For this review, take the finished solid that the model builds, in its own axes (mm). Face numbers are marked on the shaded views. A direction names the side the tool comes from. Coordinates: 2 decimals unless noted, no trailing zeros. Loops run counter-clockwise (first coordinate to the right, second up) from the corner with the lowest first, then second, coordinate; pieces in that order, holes last. Notation, with made-up numbers: (26.5, -17) - (46.5, -17) arc R31 cw to (46.5, 11) - close; hole circle Ø6 at (9.25, 79.25). An arc over 180 degrees is marked (long way). Answer as a JSON object with one key per item and string values. Group by question number.
Item 1: We need section A-A (y = 4.5). Give the boundary of the cut face in (x, z), then the cut area to 3 significant figures.
Item 2: We need section B-B (x = -5.5). Give the boundary of the cut face in (y, z), then the cut area to 3 significant figures.
Item 3: We need section D-D (x = 1). Give the boundary of the cut face in (y, z), then the cut area to 3 significant figures.
Item 4: Clearance check with flat-ended pins moving along their axes: pin 1 (0.7 mm diameter, centred on x = 6, z = 7, fed in from +Y); pin 2 (1.5 mm diameter, centred on x = -0.5, y = 18, fed in from -Z); pin 3 (4 mm diameter, centred on y = 8.5, z = 7.5, fed in from -X). State where each tip first meets the part, or that it passes through.
Item 5: Tool access review of the marked faces 5, 6, 7 and 8: name each direction out of +Z, -Z, +X, -X, +Y, -Y from which nothing blocks a thin tool from reaching the whole face with its end or side.
Item 6: To check wall thickness, follow line 1 (Z direction, x = -5.5, y = 7); line 2 (X direction, y = 7.25, z = 20.5); line 3 (Z direction, x = -1, y = 8). State the ranges of each line that lie inside material, in increasing order.
Item 7: Mouldability with a two-part tool opening along Z and no side actions: class the marked faces 1, 2, 3 and 4 as released by +Z, released by -Z, zero draft, split by the parting line, or undercut.
Item 8: We need section C-C (z = -10). Give the boundary of the cut face in (x, y), then the cut area to 3 significant figures.
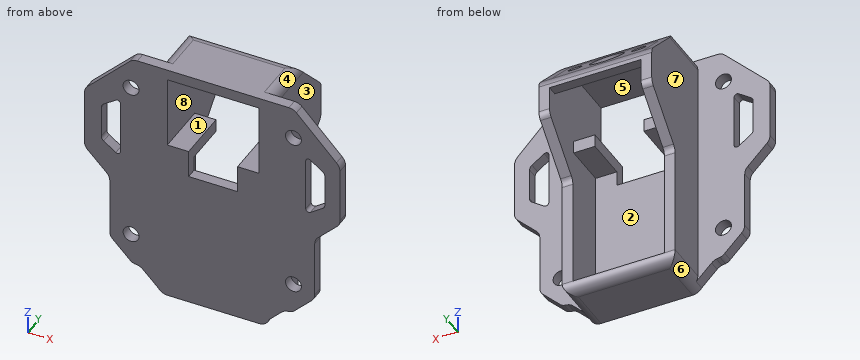
from build123d import *

# Parameters (mm, degrees)
BOSS_EXTRUDE1_DEPTH      = 2
SKETCH2_R                = 1.500000246
SKETCH2_R_2              = 1.5
CUT_EXTRUDE1_DEPTH       = 3
CUT_EXTRUDE3_DEPTH       = 3
SKETCH4_W                = 17.2
SKETCH4_H                = 42.900000423
BOSS_EXTRUDE2_DEPTH      = 16.8
BOSS_EXTRUDE2_DEPTH_BACK = 2
CUT_EXTRUDE4_DEPTH       = 35.442318281
BOSS_EXTRUDE3_REACH      = 34.758
CUT_EXTRUDE5_REACH       = 42.25
SKETCH7_R                = 3.1
SKETCH7_R_2              = 1.3
CUT_EXTRUDE6_REACH       = 4
SKETCH10_W               = 4
SKETCH10_H               = 2.4
BOSS_EXTRUDE4_DEPTH      = 8


with BuildPart() as part:
    # Sketch1 → Boss-Extrude1 (new body)
    with BuildSketch(Plane(origin=(0, 0, 0), x_dir=(1, 0, 0), z_dir=(0, 1, 0))):
        with BuildLine():
            Line((18.572356392, 15.455642083), (15.400781136, 18.627215476))
            ThreePointArc((15.400781136, 18.627215476), (15.000980559, 18.963075341), (14.510830812, 19.14306305))
            Line((14.510830812, 19.14306305), (13.829154841, 19.266075861))
            ThreePointArc((13.829154841, 19.266075861), (13.350450837, 19.465809152), (12.939209066, 19.781927984))
            Line((12.939209066, 19.781927984), (9.538270081, 23.182866969))
            ThreePointArc((9.538270081, 23.182866969), (9.061835297, 23.501210514), (8.499842151, 23.612997901))
            Line((8.499842151, 23.612997901), (-8.368205994, 23.612997901))
            ThreePointArc((-8.368205994, 23.612997901), (-9.221556491, 23.443255933), (-9.94499211, 22.959871707))
            Line((-9.94499211, 22.959871707), (-13.122935832, 19.781927984))
            ThreePointArc((-13.122935832, 19.781927984), (-13.53417801, 19.465808988), (-14.012882539, 19.266075861))
            Line((-14.012882539, 19.266075861), (-14.694557578, 19.14306305))
            ThreePointArc((-14.694557578, 19.14306305), (-15.184706626, 18.963073976), (-15.584504285, 18.627210927))
            Line((-15.584504285, 18.627210927), (-18.756076746, 15.455636602))
            ThreePointArc((-18.756076746, 15.455636602), (-19.189622668, 14.806788967), (-19.341863745, 14.041421099))
            Line((-19.341863745, 14.041421099), (-19.341863745, 3.384570997))
            ThreePointArc((-19.341863745, 3.384570997), (-19.494104434, 2.619205106), (-19.927649253, 1.970359158))
            Line((-19.927649253, 1.970359158), (-23.506077059, -1.608070511))
            ThreePointArc((-23.506077059, -1.608070511), (-23.939622981, -2.25691811), (-24.091864058, -3.022285948))
            Line((-24.091864058, -3.022285948), (-24.091864058, -13.36542942))
            ThreePointArc((-24.091864058, -13.36542942), (-23.939623268, -14.130795551), (-23.506078181, -14.779641628))
            Line((-23.506078181, -14.779641628), (-15.584504285, -22.701215524))
            ThreePointArc((-15.584504285, -22.701215524), (-14.935656966, -23.134761442), (-14.170289369, -23.287002522))
            Line((-14.170289369, -23.287002522), (14.301925526, -23.287002522))
            ThreePointArc((14.301925526, -23.287002522), (15.067293123, -23.134761442), (15.716140442, -22.701215524))
            Line((15.716140442, -22.701215524), (23.23794041, -14.862959876))
            ThreePointArc((23.23794041, -14.862959876), (23.709924747, -14.155388537), (23.90813636, -13.32826184))
            Line((23.90813636, -13.32826184), (23.90813636, -3.022286468))
            ThreePointArc((23.90813636, -3.022286468), (23.755895287, -2.25691839), (23.322349361, -1.608070511))
            Line((23.322349361, -1.608070511), (19.743924908, 1.970357668))
            ThreePointArc((19.743924908, 1.970357668), (19.310378982, 2.619205547), (19.158137909, 3.384573625))
            Line((19.158137909, 3.384573625), (19.158137909, 14.041440986))
            ThreePointArc((19.158137909, 14.041440986), (19.005898249, 14.806801151), (18.572356392, 15.455642083))
        make_face()
    extrude(amount=BOSS_EXTRUDE1_DEPTH)

    # Sketch2 → Cut-Extrude1 (cut, through all)
    with BuildSketch(Plane(origin=(0, 2, 0), x_dir=(1, 0, 0), z_dir=(0, 1, 0))):
        with Locations((-15.341864952, -17.28700247)):
            Circle(SKETCH2_R)
        with Locations((15.158137254, -17.28700247)):
            Circle(SKETCH2_R)
        with Locations((15.158137909, 13.212998804)):
            Circle(SKETCH2_R_2)
        with Locations((-15.341866539, 13.212998804)):
            Circle(SKETCH2_R_2)
    extrude(amount=-CUT_EXTRUDE1_DEPTH, mode=Mode.SUBTRACT)

    # Sketch3 → Cut-Extrude3 (cut, through all)
    with BuildSketch(Plane.XZ):
        with BuildLine():
            Line((18.332290758, 13.738059649), (20.625916482, 12.132045627))
            ThreePointArc((20.625916482, 12.132045627), (20.949257646, 11.763345693), (21.065818079, 11.287002522))
            Line((21.065818079, 11.287002522), (21.065818079, 5.287002522))
            ThreePointArc((21.065818079, 5.287002522), (20.949257646, 4.810659352), (20.625916482, 4.441959417))
            Line((20.625916482, 4.441959417), (18.332290758, 2.835945395))
            ThreePointArc((18.332290758, 2.835945395), (17.762200326, 2.798579694), (17.465818079, 3.287002522))
            Line((17.465818079, 3.287002522), (17.465818079, 13.287002522))
            ThreePointArc((17.465818079, 13.287002522), (17.762200326, 13.77542535), (18.332290758, 13.738059649))
        make_face()
        with BuildLine():
            Line((-17.334181921, 13.287002522), (-17.334181921, 3.287002522))
            ThreePointArc((-17.334181921, 3.287002522), (-17.630564169, 2.798579694), (-18.200654601, 2.835945395))
            Line((-18.200654601, 2.835945395), (-20.494280325, 4.441959417))
            ThreePointArc((-20.494280325, 4.441959417), (-20.817621489, 4.810659352), (-20.934181921, 5.287002522))
            Line((-20.934181921, 5.287002522), (-20.934181921, 11.287002522))
            ThreePointArc((-20.934181921, 11.287002522), (-20.817621489, 11.763345693), (-20.494280325, 12.132045627))
            Line((-20.494280325, 12.132045627), (-18.200654601, 13.738059649))
            ThreePointArc((-18.200654601, 13.738059649), (-17.630564169, 13.77542535), (-17.334181921, 13.287002522))
        make_face()
    extrude(amount=-CUT_EXTRUDE3_DEPTH, mode=Mode.SUBTRACT)

    # Sketch4 → Boss-Extrude2 (add, two sides)
    with BuildSketch(Plane(origin=(0, 2, 0), x_dir=(1, 0, 0), z_dir=(0, 1, 0))) as boss_extrude2_sk:
        with BuildLine():
            Line((-8.534181921, -23.287002522), (8.665818079, -23.287002522))
            ThreePointArc((8.665818079, -23.287002522), (10.080031641, -22.701216085), (10.665818079, -21.287002522))
            Line((10.665818079, -21.287002522), (10.665818079, 21.612997901))
            ThreePointArc((10.665818079, 21.612997901), (10.080031641, 23.027211463), (8.665818079, 23.612997901))
            Line((8.665818079, 23.612997901), (-8.534181921, 23.612997901))
            ThreePointArc((-8.534181921, 23.612997901), (-9.948395484, 23.027211463), (-10.534181921, 21.612997901))
            Line((-10.534181921, 21.612997901), (-10.534181921, -21.287002522))
            ThreePointArc((-10.534181921, -21.287002522), (-9.948395484, -22.701216085), (-8.534181921, -23.287002522))
        make_face()
        with Locations((0.065818079, 0.162997689)):
            Rectangle(SKETCH4_W, SKETCH4_H, mode=Mode.SUBTRACT)
    extrude(amount=BOSS_EXTRUDE2_DEPTH)
    extrude(boss_extrude2_sk.sketch, amount=-BOSS_EXTRUDE2_DEPTH_BACK)

    # Sketch5 → Cut-Extrude4 (cut, through all)
    with BuildSketch(Plane.ZY.offset(10.534181921)):
        with BuildLine():
            Line((-21.612997901, 10.3), (-1.443459743, 10.3))
            ThreePointArc((-1.443459743, 10.3), (-0.676489206, 10.452906013), (-0.026793076, 10.888243804))
            Line((-0.026793076, 10.888243804), (7.271334447, 18.211756196))
            ThreePointArc((7.271334447, 18.211756196), (7.921030577, 18.647093987), (8.688001114, 18.8))
            Line((8.688001114, 18.8), (13.837952846, 18.8))
            ThreePointArc((13.837952846, 18.8), (14.596331781, 18.650638104), (15.2414378, 18.224861392))
            Line((15.2414378, 18.224861392), (22.690487476, 10.887565848))
            ThreePointArc((22.690487476, 10.887565848), (23.131856162, 10.235048322), (23.287002522, 9.462704457))
            Line((23.287002522, 9.462704457), (23.287002522, 6.883402598))
            Line((23.287002522, 6.883402598), (26.098263888, 6.883402598))
            Line((26.098263888, 6.883402598), (26.098263888, 23.771252442))
            Line((26.098263888, 23.771252442), (-26.157105029, 23.771252442))
            Line((-26.157105029, 23.771252442), (-26.157105029, 6.5400194))
            Line((-26.157105029, 6.5400194), (-23.612997901, 6.5400194))
            Line((-23.612997901, 6.5400194), (-23.612997901, 8.3))
            ThreePointArc((-23.612997901, 8.3), (-23.027211463, 9.714213562), (-21.612997901, 10.3))
        make_face()
    extrude(amount=-CUT_EXTRUDE4_DEPTH, mode=Mode.SUBTRACT)

    # Sketch6 → Boss-Extrude3 (add, up to next)
    with BuildSketch(Plane.ZY.offset(-8.665818079), mode=Mode.PRIVATE) as boss_extrude3_sk1:
        with BuildLine():
            Line((21.287002522, 12.269995063), (15.2414378, 18.224861392))
            ThreePointArc((15.2414378, 18.224861392), (14.596331781, 18.650638104), (13.837952846, 18.8))
            Line((13.837952846, 18.8), (13.034792435, 18.8))
            Line((13.034792435, 18.8), (13.034792435, 16.889288371))
            Line((13.034792435, 16.889288371), (21.313555812, 8.73472688))
            Line((21.313555812, 8.73472688), (23.287002522, 8.73472688))
            Line((23.287002522, 8.73472688), (23.287002522, 9.462704457))
            ThreePointArc((23.287002522, 9.462704457), (23.131856162, 10.235048322), (22.690487476, 10.887565848))
            Line((22.690487476, 10.887565848), (21.287002522, 12.269995063))
        make_face()
    boss_extrude3_tool1 = extrude(boss_extrude3_sk1.sketch, amount=BOSS_EXTRUDE3_REACH, mode=Mode.PRIVATE) - part.part
    add(boss_extrude3_tool1.solids().sort_by_distance((8.665818, 13.686528, 18.07587))[0])

    # Sketch7 → Cut-Extrude5 (cut, up to next)
    with BuildSketch(Plane(origin=(0, 16.870013343, 16.6169215), x_dir=(1, 0, 0), z_dir=(0, 0.712430696, 0.701742477)), mode=Mode.PRIVATE) as cut_extrude5_sk1:
        with Locations((0.065818079, -3.297220561)):
            Circle(SKETCH7_R)
    cut_extrude5_tool1 = extrude(cut_extrude5_sk1.sketch, amount=-CUT_EXTRUDE5_REACH, mode=Mode.PRIVATE) & part.part
    add(cut_extrude5_tool1.solids().sort_by_distance((0.065818, 14.556214, 18.965963))[0], mode=Mode.SUBTRACT)
    # Sketch7 → Cut-Extrude5 (cut, up to next)
    with BuildSketch(Plane(origin=(0, 16.870013343, 16.6169215), x_dir=(1, 0, 0), z_dir=(0, 0.712430696, 0.701742477)), mode=Mode.PRIVATE) as cut_extrude5_sk2:
        with Locations((6.065818079, -3.297220561)):
            Circle(SKETCH7_R_2)
    cut_extrude5_tool2 = extrude(cut_extrude5_sk2.sketch, amount=-CUT_EXTRUDE5_REACH, mode=Mode.PRIVATE) & part.part
    add(cut_extrude5_tool2.solids().sort_by_distance((6.065818, 14.556214, 18.965963))[0], mode=Mode.SUBTRACT)
    # Sketch7 → Cut-Extrude5 (cut, up to next)
    with BuildSketch(Plane(origin=(0, 16.870013343, 16.6169215), x_dir=(1, 0, 0), z_dir=(0, 0.712430696, 0.701742477)), mode=Mode.PRIVATE) as cut_extrude5_sk3:
        with Locations((-5.934181921, -3.297220561)):
            Circle(SKETCH7_R_2)
    cut_extrude5_tool3 = extrude(cut_extrude5_sk3.sketch, amount=-CUT_EXTRUDE5_REACH, mode=Mode.PRIVATE) & part.part
    add(cut_extrude5_tool3.solids().sort_by_distance((-5.934182, 14.556214, 18.965963))[0], mode=Mode.SUBTRACT)

    # Sketch9 → Cut-Extrude6 (cut, up to next)
    with BuildSketch(Plane(origin=(0, 2, 0), x_dir=(1, 0, 0), z_dir=(0, 1, 0)), mode=Mode.PRIVATE) as cut_extrude6_sk1:
        Polygon((-8.534181921, -21.287002522), (8.665818079, -21.287002522), (8.665818079, -7.687002522), (4.665818079, -7.687002522), (4.665818079, -2.492093964), (-4.534181921, -2.492093964), (-4.534181921, -7.687002522), (-8.534181921, -7.687002522), align=None)
    cut_extrude6_tool1 = extrude(cut_extrude6_sk1.sketch, amount=-CUT_EXTRUDE6_REACH, mode=Mode.PRIVATE) & part.part
    add(cut_extrude6_tool1.solids().sort_by_distance((0.065818, 2, 12.892707))[0], mode=Mode.SUBTRACT)

    # Sketch10 → Boss-Extrude4 (add)
    with BuildSketch(Plane(origin=(0, 2, 0), x_dir=(1, 0, 0), z_dir=(0, 1, 0))):
        with Locations((6.665818079, -6.487002522)):
            Rectangle(SKETCH10_W, SKETCH10_H)
        with Locations((-6.534181921, -6.487002522)):
            Rectangle(SKETCH10_W, SKETCH10_H)
    extrude(amount=BOSS_EXTRUDE4_DEPTH)


solid = part.part
Check sheet entries:
{
 "1": {"outline": "(-10.53, -21.61) arc R2 ccw to (-8.53, -23.61) - (8.67, -23.61) arc R2 ccw to (10.67, -21.61) - (10.67, 21.29) arc R2 ccw to (8.67, 23.29) - (-8.53, 23.29) arc R2 ccw to (-10.53, 21.29) - close; hole (-8.53, -21.61) - (8.67, -21.61) - (8.67, 5.29) - (4.67, 5.29) - (4.67, 7.69) - (8.67, 7.69) - (8.67, 21.29) - (-8.53, 21.29) - (-8.53, 7.69) - (-4.53, 7.69) - (-4.53, 5.29) - (-8.53, 5.29) - close", "area": "272 mm2"},
 "2": {"outline": "(0, -23.61) - (8.3, -23.61) arc R2 ccw to (10.3, -21.61) - (2, -21.61) - (2, 5.29) - (10, 5.29) - (10, 7.69) - (0, 7.69) - close; (0, 21.29) - (8.76, 21.29) - (11.92, 18.08) - (13.7, 19.84) - (10.89, 22.69) arc R2 ccw to (9.46, 23.29) - (0, 23.29) - close; (13.64, 16.34) - (16.89, 13.03) - (18.8, 13.03) - (18.8, 13.84) arc R2 ccw to (18.22, 15.24) - (15.42, 18.09) - close", "area": "141 mm2"},
 "3": {"outline": "(0, -23.61) - (8.3, -23.61) arc R2 ccw to (10.3, -21.61) - (2, -21.61) - (2, 2.49) - (0, 2.49) - close; (0, 21.29) - (8.76, 21.29) - (10.7, 19.32) - (12.48, 21.07) - (10.89, 22.69) arc R2 ccw to (9.46, 23.29) - (0, 23.29) - close; (14.85, 15.11) - (16.89, 13.03) - (18.8, 13.03) - (18.8, 13.84) arc R2 ccw to (18.22, 15.24) - (16.63, 16.86) - close", "area": "103 mm2"},
 "4": {"pin 1": "stops at y = 10", "pin 2": "stops at z = 13.03", "pin 3": "stops at x = -10.53"},
 "5": {"face 5": "-Y", "face 6": "-Z, -X, +Y", "face 7": "+Z, -Z, -X, +Y", "face 8": "none"},
 "6": {"line 1": "z = -23.61 to -21.61, 5.29 to 7.69, 21.29 to 23.29", "line 2": "x = -10.53 to -8.53, 8.67 to 10.67", "line 3": "z = -23.61 to -21.61, 21.29 to 23.29"},
 "7": {"face 1": "undercut", "face 2": "undercut", "face 3": "zero draft", "face 4": "released by +Z"},
 "8": {"outline": "(-19.34, 0) - (19.16, 0) - (19.16, 2) - (10.67, 2) - (10.67, 10.3) - (8.67, 10.3) - (8.67, 2) - (-8.53, 2) - (-8.53, 10.3) - (-10.53, 10.3) - (-10.53, 2) - (-19.34, 2) - close", "area": "110 mm2"}
}
